Autodesk Inventor part; units mm, degrees
ref_plane "YZ Plane" through (0, 0, 0) normal (1, 0, 0) x (0, 1, 0)
ref_plane "XZ Plane" through (0, 0, 0) normal (0, 1, 0) x (-1, 0, 0)
ref_plane "XY Plane" through (0, 0, 0) normal (0, 0, 1) x (1, 0, 0)
sketch "Sketch1" plane through (0, 0, 0) normal (0, 0, 1) x (1, 0, 0)
  circle A0 centre (0, 0) radius 2.5
  line L0 (-9.9932, 4.515) -> (-7.9864, 3.0135)
  line L1 (-7.486, 6.0081) -> (-7.2469, 6.008)
  line L2 (-6.8934, 5.8613) -> (-4.8771, 3.8419)
  arc A1 (-6.8934, 5.8613) -> (-7.2469, 6.008) centre (-7.2472, 5.508) ccw
  circle A2 centre (0, 0) radius 2.5
  line L3 (-9.9932, 4.515) -> (-9.9932, 9.9932)
  line L4 (-7.9864, 3.0135) -> (-7.9864, 5.5081)
  arc A3 (-7.486, 6.0081) -> (-7.9864, 5.5081) centre (-7.4864, 5.5081) ccw
  line L5 (-4, 1.7222) -> (-4, 0)
  line L6 (-9.9932, -4.515) -> (-7.9864, -3.0135)
  line L7 (-6.8934, -5.8613) -> (-4.8771, -3.8419)
  arc A4 (-7.2469, -6.008) -> (-6.8934, -5.8613) centre (-7.2472, -5.508) ccw
  line L8 (-7.486, -6.0081) -> (-7.2469, -6.008)
  line L9 (-9.9932, -4.515) -> (-9.9932, -9.9932)
  line L10 (-7.9864, -3.0135) -> (-7.9864, -5.5081)
  arc A5 (-7.9864, -5.5081) -> (-7.486, -6.0081) centre (-7.4864, -5.5081) ccw
  line L11 (-4, -1.7222) -> (-4, 0)
  line L12 (9.9932, 4.515) -> (7.9864, 3.0135)
  line L13 (6.8934, 5.8613) -> (4.8771, 3.8419)
  arc A6 (7.2469, 6.008) -> (6.8934, 5.8613) centre (7.2472, 5.508) ccw
  line L14 (7.486, 6.0081) -> (7.2469, 6.008)
  line L15 (9.9932, 4.515) -> (9.9932, 9.9932)
  line L16 (7.9864, 3.0135) -> (7.9864, 5.5081)
  arc A7 (7.9864, 5.5081) -> (7.486, 6.0081) centre (7.4864, 5.5081) ccw
  line L17 (4, 1.7222) -> (4, 0)
  line L18 (9.9932, -4.515) -> (7.9864, -3.0135)
  line L19 (6.8934, -5.8613) -> (4.8771, -3.8419)
  arc A8 (6.8934, -5.8613) -> (7.2469, -6.008) centre (7.2472, -5.508) ccw
  line L20 (7.486, -6.0081) -> (7.2469, -6.008)
  line L21 (9.9932, -4.515) -> (9.9932, -9.9932)
  line L22 (7.9864, -3.0135) -> (7.9864, -5.5081)
  arc A9 (7.486, -6.0081) -> (7.9864, -5.5081) centre (7.4864, -5.5081) ccw
  line L23 (4, -1.7222) -> (4, 0)
  circle A10 centre (0, 0) radius 2.5
  line L24 (-4.515, -9.9932) -> (-3.0135, -7.9864)
  line L25 (-5.8613, -6.8934) -> (-3.8419, -4.8771)
  arc A11 (-5.8613, -6.8934) -> (-6.008, -7.2469) centre (-5.508, -7.2472) ccw
  line L26 (-6.0081, -7.486) -> (-6.008, -7.2469)
  circle A12 centre (0, 0) radius 2.5
  line L27 (-4.515, -9.9932) -> (-9.9932, -9.9932)
  line L28 (-3.0135, -7.9864) -> (-5.5081, -7.9864)
  arc A13 (-6.0081, -7.486) -> (-5.5081, -7.9864) centre (-5.5081, -7.4864) ccw
  line L29 (-1.7222, -4) -> (0, -4)
  line L30 (4.515, -9.9932) -> (3.0135, -7.9864)
  line L31 (5.8613, -6.8934) -> (3.8419, -4.8771)
  arc A14 (6.008, -7.2469) -> (5.8613, -6.8934) centre (5.508, -7.2472) ccw
  line L32 (6.0081, -7.486) -> (6.008, -7.2469)
  line L33 (4.515, -9.9932) -> (9.9932, -9.9932)
  line L34 (3.0135, -7.9864) -> (5.5081, -7.9864)
  arc A15 (5.5081, -7.9864) -> (6.0081, -7.486) centre (5.5081, -7.4864) ccw
  line L35 (1.7222, -4) -> (0, -4)
  line L36 (-1.7222, 4) -> (0, 4)
  line L37 (1.7222, 4) -> (0, 4)
  line L38 (5.8613, 6.8934) -> (3.8419, 4.8771)
  arc A16 (5.8613, 6.8934) -> (6.008, 7.2469) centre (5.508, 7.2472) ccw
  line L39 (6.0081, 7.486) -> (6.008, 7.2469)
  line L40 (3.0135, 7.9864) -> (5.5081, 7.9864)
  arc A17 (6.0081, 7.486) -> (5.5081, 7.9864) centre (5.5081, 7.4864) ccw
  line L41 (4.515, 9.9932) -> (3.0135, 7.9864)
  line L42 (4.515, 9.9932) -> (9.9932, 9.9932)
  line L43 (-5.8613, 6.8934) -> (-3.8419, 4.8771)
  arc A18 (-6.008, 7.2469) -> (-5.8613, 6.8934) centre (-5.508, 7.2472) ccw
  line L44 (-6.0081, 7.486) -> (-6.008, 7.2469)
  line L45 (-3.0135, 7.9864) -> (-5.5081, 7.9864)
  arc A19 (-5.5081, 7.9864) -> (-6.0081, 7.486) centre (-5.5081, 7.4864) ccw
  line L46 (-4.515, 9.9932) -> (-3.0135, 7.9864)
  line L47 (-4.515, 9.9932) -> (-9.9932, 9.9932)
  arc A20 (1.7222, 4) -> (3.8419, 4.8771) centre (1.7222, 7) ccw
  arc A21 (-3.8419, 4.8771) -> (-1.7222, 4) centre (-1.7222, 7) ccw
  arc A22 (-4, 1.7222) -> (-4.8771, 3.8419) centre (-7, 1.7222) ccw
  arc A23 (-4.8771, -3.8419) -> (-4, -1.7222) centre (-7, -1.7222) ccw
  arc A24 (-1.7222, -4) -> (-3.8419, -4.8771) centre (-1.7222, -7) ccw
  arc A25 (3.8419, -4.8771) -> (1.7222, -4) centre (1.7222, -7) ccw
  arc A26 (4, -1.7222) -> (4.8771, -3.8419) centre (7, -1.7222) ccw
  arc A27 (4.8771, 3.8419) -> (4, 1.7222) centre (7, 1.7222) ccw
  point P0 (-7.9864, 6.0085)
  point P1 (-7.9864, -6.0085)
  point P2 (7.9864, 6.0085)
  point P3 (7.9864, -6.0085)
  point P4 (-6.0085, -7.9864)
  point P5 (6.0085, -7.9864)
  point P6 (6.0085, 7.9864)
  point P7 (-6.0085, 7.9864)
extrude "Extrusion9" add sketch "Sketch1" along normal blind 288.925
properties part number "20mm_V-Rail_Extrusion Template" material "6105-T5 Aluminum"
Can you work these out from the model? Positions are in its coordinate system, mm. Give positions to 0.01 mm unless a question says otherwise; leave off trailing zeros. Use a Markdown table: item, result. Add a question column.
Item 1: Will these pins go through, and if not, where does the flat tip stop? pin 1 (0.7 mm diameter, centred on y = 4, z = 121.5, fed in from +X); pin 2 (1 mm diameter, centred on y = -0.5, z = 151.5, fed in from +X); pin 3 (3 mm diameter, centred on x = 0, z = 182.5, fed in from -Y).
Item 2: If I drill on L1, parallel to X at y = 7.5, z = 108.5; L2, parallel to X at y = -6.5, z = 119; L3, parallel to Y at x = 0, z = 174, over which ranges is the centre line in solid material (lowest first)? Write a range as [from, to].
Item 3: We'd pull the mould along X, two halves only. Please class faces 1 (the flat face through (9.993, -7, 142)), 2 (the cylindrical face through (-0.54, 2.44, 142.44)), 3 (the flat face through (7, 9.993, 142)): +X half, -X half, draft (parallel to the pull), parting line (faces both ways), or undercut.
Answer sheet:
| question | item | result |
|---|---|---|
| 1 | pin 1 | stops at x = 9.77 |
| 1 | pin 2 | stops at x = 4 |
| 1 | pin 3 | stops at y = -4 |
| 2 | L1 | x = [-9.99, -6.01], [6.01, 9.99] |
| 2 | L2 | x = [-9.99, -5.47], [5.47, 9.99] |
| 2 | L3 | y = [-4, -2.5], [2.5, 4] |
| 3 | face 1 | +X half |
| 3 | face 2 | undercut |
| 3 | face 3 | draft |
